The drawing under review shows one solid part. Ordinate dimensions are in mm from its lowest x, y, z. A direction names the side the tool comes from. Give positions to 0.01 mm unless a question says otherwise; leave off trailing zeros. Write each loop counter-clockwise with the first axis right and the second up, starting at its lowest first coordinate (ties: lowest second). Pieces come first, ordered by that corner, then holes. Notation, with made-up numbers: (49.25, 45.5) -> (84.25, 45.5) arc R23 ccw to (84.25, 72.5) -> close; hole circle Ø3 at (79.5, 11). An arc over 180 degrees is marked (long way). Put each result on its own line as item: value. Start each with the question number.
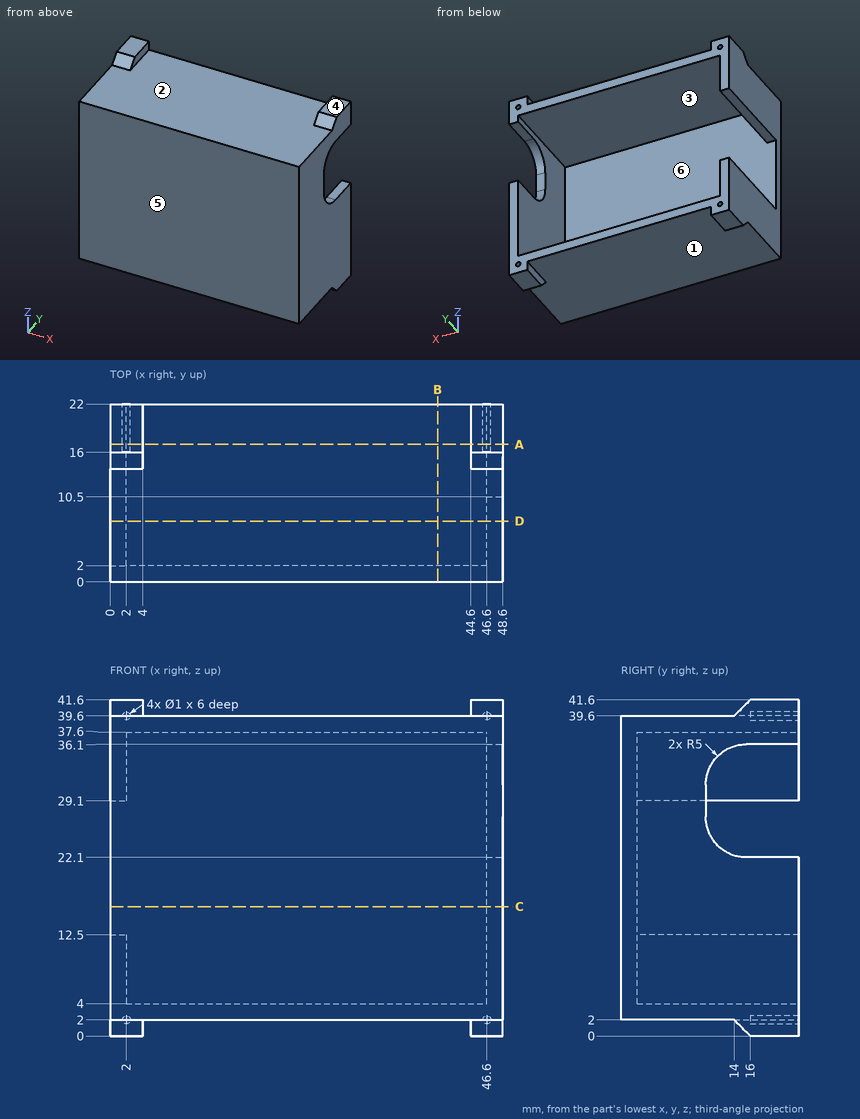
Q1. Take a section at C-C on z = 16. Give the boundary of the cut face in (x, y), then the cut area to 3 significant figures.
Q2. To check wall thickness, follow probe 1 along Z at (x, y) = (16, 16.5); probe 2 along X at (y, z) = (3.5, 10); probe 3 along Y at (x, z) = (27, 30). State the ranges of each line that lie inside material, in increasing order. Write a range as from..to.
Q3. Take a section at A-A on y = 17. Give the boundary of the cut face in (x, z).
Q4. Machinability: for the marked faces 1, 2 and 3, which of the approach directions +Z, -Z, +X, -X, +Y, -Y give a long, thin tool a straight path to every point of the face, cutting with its end or side? Answer none if there is none.
Q5. Take a section at B-B on x = 40.5. Give the boundary of the cut face in (y, z).
Q6. Take a section at D-D on y = 7.5. Give the boundary of the cut face in (x, z), then the cut area to 3 significant figures.
Q7. Mouldability with a two-part tool opening along Z and no side actions: class the marked faces 4, 5 and 6 as +Z half, -Z half, draft (parallel to the pull), parting line (faces both ways), or undercut.
Q8. For pin 1 (12 mm diameter, centred on x = 35, y = 4, fed in from -Z); pin 2 (5 mm diameter, centred on x = 15.5, z = 29, fed in from -Y); pin 3 (5 mm diameter, centred on x = 30.5, y = 16, fed in from +Z); pin 4 (2 mm diameter, centred on x = 47.5, z = 30, fed in from +Y), all flat-tipped, find the tip position at first contact; note any pin that passes through.
Result:
1. outline: (0, 0) -> (48.6, 0) -> (48.6, 22) -> (46.6, 22) -> (46.6, 2) -> (0, 2) -> close
1. area: 137 mm^2
2. probe 1: z = 2..4, 37.6..39.6
2. probe 2: x = 0..2, 46.6..48.6
2. probe 3: y = 0..2
3. outline: (0, 0) -> (4, 0) -> (4, 2) -> (44.6, 2) -> (44.6, 0) -> (48.6, 0) -> (48.6, 22.1) -> (46.6, 22.1) -> (46.6, 4) -> (2, 4) -> (2, 12.5) -> (0, 12.5) -> close; (0, 29.1) -> (2, 29.1) -> (2, 37.6) -> (46.6, 37.6) -> (46.6, 36.1) -> (48.6, 36.1) -> (48.6, 41.6) -> (44.6, 41.6) -> (44.6, 39.6) -> (4, 39.6) -> (4, 41.6) -> (0, 41.6) -> close; hole circle Ø1 at (2, 2); hole circle Ø1 at (2, 39.6); hole circle Ø1 at (46.6, 2); hole circle Ø1 at (46.6, 39.6)
4. face 1: -Z, -Y
4. face 2: +Z, -Y
4. face 3: +Y
5. outline: (0, 2) -> (22, 2) -> (22, 4) -> (2, 4) -> (2, 37.6) -> (22, 37.6) -> (22, 39.6) -> (0, 39.6) -> close
6. outline: (0, 2) -> (48.6, 2) -> (48.6, 39.6) -> (0, 39.6) -> (0, 29.1) -> (2, 29.1) -> (2, 37.6) -> (46.6, 37.6) -> (46.6, 4) -> (2, 4) -> (2, 12.5) -> (0, 12.5) -> close
6. area: 296 mm^2
7. face 4: +Z half
7. face 5: draft
7. face 6: undercut
8. pin 1: stops at z = 2
8. pin 2: stops at y = 0
8. pin 3: stops at z = 39.6
8. pin 4: stops at y = 10.5
